```python
from build123d import *

# Parameters (mm, degrees)
SKETCH1_R           = 1.6
BOSS_EXTRUDE1_DEPTH = 8
SKETCH2_W           = 9
SKETCH2_H           = 8.199711987
CUT_EXTRUDE1_DEPTH  = 8
BOSS_EXTRUDE2_DEPTH = 6
SKETCH4_R           = 1.6
BOSS_EXTRUDE3_DEPTH = 8


with BuildPart() as part:
    # Sketch1 → Boss-Extrude1 (new body)
    with BuildSketch(Plane.XY):
        with BuildLine():
            Line((-0.5, 3), (15.5, 3))
            ThreePointArc((15.5, 3), (17.267766953, 2.267766953), (18, 0.5))
            Line((18, 0.5), (18, -0.5))
            ThreePointArc((18, -0.5), (17.267766953, -2.267766953), (15.5, -3))
            Line((15.5, -3), (-0.5, -3))
            ThreePointArc((-0.5, -3), (-2.267766953, -2.267766953), (-3, -0.5))
            Line((-3, -0.5), (-3, 0.5))
            ThreePointArc((-3, 0.5), (-2.267766953, 2.267766953), (-0.5, 3))
        make_face()
        Circle(SKETCH1_R, mode=Mode.SUBTRACT)
        with Locations((15, 0)):
            Circle(SKETCH1_R, mode=Mode.SUBTRACT)
    extrude(amount=BOSS_EXTRUDE1_DEPTH)

    # Sketch2 → Cut-Extrude1 (cut)
    with BuildSketch(Plane.XZ.offset(3)):
        with Locations((7.5, 6.099855994)):
            Rectangle(SKETCH2_W, SKETCH2_H)
    extrude(amount=-CUT_EXTRUDE1_DEPTH, mode=Mode.SUBTRACT)

    # Sketch3 → Boss-Extrude2 (add)
    with BuildSketch(Plane.XZ.offset(3)):
        Polygon((3.257359313, 2), (7.5, 6.242640687), (11.742640687, 2), align=None)
    extrude(amount=-BOSS_EXTRUDE2_DEPTH)

    # Sketch4 → Boss-Extrude3 (add)
    with BuildSketch(Plane(origin=(0, 0, 0), x_dir=(-1, 0, 0), z_dir=(0, 0, -1))):
        with BuildLine():
            Line((15.5, 3), (0.5, 3))
            ThreePointArc((0.5, 3), (2.267766953, 2.267766953), (3, 0.5))
            Line((3, 0.5), (3, -0.5))
            ThreePointArc((3, -0.5), (2.267766953, -2.267766953), (0.5, -3))
            Line((0.5, -3), (15.5, -3))
            ThreePointArc((15.5, -3), (17.267766953, -2.267766953), (18, -0.5))
            Line((18, -0.5), (18, 0.5))
            ThreePointArc((18, 0.5), (17.267766953, 2.267766953), (15.5, 3))
        make_face()
        with Locations((7.5, 0)):
            Circle(SKETCH4_R, mode=Mode.SUBTRACT)
        with Locations((15, 0)):
            Circle(SKETCH4_R, mode=Mode.SUBTRACT)
        with BuildLine():
            ThreePointArc((-18, 0.5), (-17.267766953, 2.267766953), (-15.5, 3))
            Line((-15.5, 3), (-30.5, 3))
            ThreePointArc((-30.5, 3), (-32.267766953, 2.267766953), (-33, 0.5))
            Line((-33, 0.5), (-33, -0.5))
            ThreePointArc((-33, -0.5), (-32.267766953, -2.267766953), (-30.5, -3))
            Line((-30.5, -3), (-15.5, -3))
            ThreePointArc((-15.5, -3), (-17.267766953, -2.267766953), (-18, -0.5))
            Line((-18, -0.5), (-18, 0.5))
        make_face()
        with Locations((-30, 0)):
            Circle(SKETCH4_R, mode=Mode.SUBTRACT)
        with Locations((-22.5, 0)):
            Circle(SKETCH4_R, mode=Mode.SUBTRACT)
    extrude(amount=-BOSS_EXTRUDE3_DEPTH)


solid = part.part
```
Geometry check sheet. Reference: the model listing, model coordinates, mm. A direction names the side the tool comes from. Give positions to 0.01 mm unless a question says otherwise; leave off trailing zeros. Write each loop counter-clockwise with the first axis right and the second up, starting at its lowest first coordinate (ties: lowest second). Pieces come first, ordered by that corner, then holes.
1) Section check D-D, the plane y = -2.5. Record the boundary of the cut face in (x, z).
2) Gauge pin test, flat end, axial feed: pin 1 (3 mm diameter, centred on x = 30, y = 0, fed in from -Z). Record the tip position at first contact, or that the pin passes through.
3) Section check A-A, the plane x = 22.5. Record the boundary of the cut face in (y, z).
4) Access from +Z, -Z, +X, -X, +Y, -Y to the whole of each face (thin tool, end or side, straight path). Record for faces 4 (the flat face through (12, 0, 5)), 5 (the cylindrical face through (20.974, 0.481, 3.944)).
5) Release check for a two-part mould opening along X. For faces 1 (the cylindrical face through (-17.287, 2.248, 3.944)), 2 (the cylindrical face through (-1.27, -0.97, 3.94)), 3 (the cylindrical face through (32.287, -2.248, 3.944)) record: pulls with the +X half, pulls with the -X half, needs draft (parallel to the pull), parting line crosses it, or undercut.
6) Material ranges on L1, parallel to Y at x = 30, z = 6; L2, parallel to X at y = 2.3, z = 3; L3, parallel to X at y = -1.9, z = 5, recorded low to high.
7) Section check B-B, the plane z = 2.5. State how many separate pieces and enclosed holes the cut face has, and give its area (3 significant figures).
Computed:
1. outline: (-17, 0) - (32, 0) - (32, 8) - (12, 8) - (12, 2) - (11.74, 2) - (7.5, 6.24) - (3.26, 2) - (3, 2) - (3, 8) - (-17, 8) - close
2. pin 1: passes through
3. outline: (-3, 0) - (-1.6, 0) - (-1.6, 8) - (-3, 8) - close; (1.6, 0) - (3, 0) - (3, 8) - (1.6, 8) - close
4. face 4: +Z, +Y, -Y
4. face 5: +Z, -Z
5. face 1: pulls with the -X half
5. face 2: undercut
5. face 3: pulls with the +X half
6. L1: y = -3 to -1.6, 1.6 to 3
6. L2: x = -17.23 to 3, 4.26 to 10.74, 12 to 32.23
6. L3: x = -17.57 to 3, 6.26 to 8.74, 12 to 32.57
7. separate pieces: 3
7. enclosed holes: 6
7. area: 243 mm2
